Geometry check sheet. Reference: the model listing, model coordinates, mm. A direction names the side the tool comes from. Give positions to 0.01 mm unless a question says otherwise; leave off trailing zeros. Order: outer loops, then holes, each group sorted by start corner. A loop starts at its lowest first (then second) coordinate and runs counter-clockwise, first axis right, second up. Notation, with made-up numbers: M 36.5,85.25 L 78.5,85.25 A9 cw 78.5,94.25 Z; hole C 3.25,68.5 d2. An arc over 180 degrees is marked long. Answer as CSV lines item,"result". Start each with the question number.
```python
from build123d import *

# Parameters (mm, degrees)
SKETCH_1_W               = 28
SKETCH_1_H               = 64
EXTRUDE_1_DEPTH          = 74
SKETCH_2_R               = 2.5
CUT_EXTRUDE_1_DEPTH      = 10
CUT_EXTRUDE_2_DEPTH      = 99.833192805
CUT_EXTRUDE_2_DEPTH_BACK = 99.833192805
SKETCH_3_W               = 54
SKETCH_3_H               = 40
EXTRUDE_2_DEPTH          = 80
SKETCH_6_R               = 10.5
CUT_EXTRUDE_3_DEPTH      = 123.719191653
SKETCH_11_W              = 28
SKETCH_11_H              = 5
SKETCH_11_H_2            = 4
EXTRUDE_5_DEPTH          = 67
SKETCH_12_R              = 2
CUT_EXTRUDE_8_DEPTH      = 122.231184107
CHAMFER_1_SIZE           = 10
SKETCH_13_R              = 10.5
SKETCH_13_R_2            = 9.5
EXTRUDE_6_DEPTH          = 25
SKETCH_14_R              = 2
CUT_EXTRUDE_9_DEPTH      = 119.894911582
SKETCH_15_R              = 2
CUT_EXTRUDE_10_DEPTH     = 122.342490596
CHAMFER_2_SIZE           = 3


with BuildPart() as part:
    # 草图1 → 凸台-拉伸1 (new body)
    with BuildSketch(Plane.XY):
        with Locations((0, 32)):
            Rectangle(SKETCH_1_W, SKETCH_1_H)
    extrude(amount=EXTRUDE_1_DEPTH)

    # 草图2 → 切除-拉伸1 (cut)
    with BuildSketch(Plane.XY.offset(74)):
        with Locations((-8, 58)):
            Circle(SKETCH_2_R)
        with Locations((8, 58)):
            Circle(SKETCH_2_R)
        with Locations((-8, 6)):
            Circle(SKETCH_2_R)
        with Locations((8, 6)):
            Circle(SKETCH_2_R)
    extrude(amount=-CUT_EXTRUDE_1_DEPTH, mode=Mode.SUBTRACT)

    # 草图3 → 切除-拉伸2 (cut, two sides: drawn at the far end of the back side and taken through both)
    with BuildSketch(Plane(origin=(0, 0, 0), x_dir=(0, 0, -1), z_dir=(1, 0, 0)).offset(-CUT_EXTRUDE_2_DEPTH_BACK)):
        with Locations((-37, 32)):
            Rectangle(SKETCH_3_W, SKETCH_3_H)
    extrude(amount=CUT_EXTRUDE_2_DEPTH + CUT_EXTRUDE_2_DEPTH_BACK, mode=Mode.SUBTRACT)

    # 草图4 → 凸台-拉伸2 (add)
    with BuildSketch(Plane(origin=(0, 0, 37), x_dir=(-1, 0, 0), z_dir=(0, 0, -1))):
        with BuildLine():
            Line((-14, 2), (14, 2))
            Line((14, 2), (14, -14))
            ThreePointArc((14, -14), (0, -28), (-14, -14))
            Line((-14, -14), (-14, 2))
        make_face()
        with BuildLine():
            Line((14, 62), (14, 78))
            ThreePointArc((14, 78), (0, 92), (-14, 78))
            Line((-14, 78), (-14, 62))
            Line((-14, 62), (14, 62))
        make_face()
    extrude(amount=EXTRUDE_2_DEPTH)

    # 草图6 → 切除-拉伸3 (cut, through all)
    with BuildSketch(Plane(origin=(0, 0, 37), x_dir=(-1, 0, 0), z_dir=(0, 0, -1))):
        with Locations((0, -14)):
            Circle(SKETCH_6_R)
        with Locations(Location((0, 78, 0), (0, 0, 180))):
            Circle(SKETCH_6_R)
    extrude(amount=CUT_EXTRUDE_3_DEPTH, mode=Mode.SUBTRACT)

    # 草图11 → 凸台-拉伸5 (add)
    with BuildSketch(Plane(origin=(0, 0, 0), x_dir=(-1, 0, 0), z_dir=(0, 0, -1))):
        with Locations((0, 64.5)):
            Rectangle(SKETCH_11_W, SKETCH_11_H)
        Rectangle(SKETCH_11_W, SKETCH_11_H_2)
    extrude(amount=EXTRUDE_5_DEPTH)

    # 草图12 → 切除-拉伸8 (cut, through all)
    with BuildSketch(Plane(origin=(0, 67, 0), x_dir=(1, 0, 0), z_dir=(0, 1, 0))):
        with Locations(Location((-9, 62, 0), (0, 0, 270))):
            Circle(SKETCH_12_R)
        with Locations(Location((9, 62, 0), (0, 0, 270))):
            Circle(SKETCH_12_R)
    extrude(amount=-CUT_EXTRUDE_8_DEPTH, mode=Mode.SUBTRACT)

    # 倒角1
    chamfer_1_edges = [part.edges().sort_by_distance(p)[0] for p in [
        (0, 62, 0),
        (0, 2, 0),
    ]]
    chamfer(chamfer_1_edges, length=CHAMFER_1_SIZE)

    # 草图13 → 凸台-拉伸6 (add, symmetric)
    # profile 1 of 2: a face of its own
    with BuildSketch(Plane.XY.offset(-3)):
        with Locations((0, 78)):
            Circle(SKETCH_13_R)
        with Locations((0, 78)):
            Circle(SKETCH_13_R_2, mode=Mode.SUBTRACT)
    # profile 2 of 2: a face of its own
    with BuildSketch(Plane.XY.offset(-3)):
        with Locations(Location((0, -14, 0), (0, 0, 180))):
            Circle(SKETCH_13_R)
        with Locations(Location((0, -14, 0), (0, 0, 180))):
            Circle(SKETCH_13_R_2, mode=Mode.SUBTRACT)
    extrude(amount=EXTRUDE_6_DEPTH, both=True)

    # 草图14 → 切除-拉伸9 (cut, through all)
    with BuildSketch(Plane(origin=(0, 0, 0), x_dir=(0, 0, -1), z_dir=(1, 0, 0))):
        with Locations((-29, 78)):
            Circle(SKETCH_14_R)
        with Locations((35, 78)):
            Circle(SKETCH_14_R)
        with Locations((35, -14)):
            Circle(SKETCH_14_R)
        with Locations((-29, -14)):
            Circle(SKETCH_14_R)
    extrude(amount=-CUT_EXTRUDE_9_DEPTH, mode=Mode.SUBTRACT)

    # 草图15 → 切除-拉伸10 (cut, through all)
    with BuildSketch(Plane.ZY.offset(14)):
        with Locations(Location((34, 58, 0), (0, 0, 270))):
            Circle(SKETCH_15_R)
    extrude(amount=-CUT_EXTRUDE_10_DEPTH, mode=Mode.SUBTRACT)

    # 倒角2
    chamfer_2_edges = [part.edges().sort_by_distance(p)[0] for p in [
        (-9, -2, -64),
        (-9, 67, -64),
        (9, -2, -64),
        (9, 67, -64),
    ]]
    chamfer(chamfer_2_edges, length=CHAMFER_2_SIZE - 0.0001)  # a hair under: the kernel refuses the full size


solid = part.part
```
Item 1: Section check A-A on z = 25.5. Record the boundary of the cut face in (x, y), then the cut area to 3 significant figures.
Item 2: Depth check by flat-ended pin: pin 1 Ø6 at (x, z) = (10.5, 32) entering from -Y; pin 2 Ø15 at (x, y) = (0, 78) entering from -Z; pin 3 Ø14 at (x, y) = (-5, 23) entering from -Z; pin 4 Ø8.5 at (x, z) = (2.5, 49.5) entering from +Y. Enter the tip coordinate at first touch or a pass-through.
Item 3: Section check D-D on x = 0. Give the number of separate pieces and of enclosed holes in the cut face, then the cut area to 3 significant figures.
Item 4: Draft check along Y on faces 4 (the face through (0, -3, -43)), 5 (the face through (0, 92, -2)), 6 (the face through (-12.128, 78.601, 27.092)). Enter one of: pulls with the +Y half, pulls with the -Y half, needs draft (parallel to the pull), parting line crosses it, or undercut.
Item 5: Section check B-B on y = 32. Record the boundary of the cut face in (x, z).
Item 6: Access from +Z, -Z, +X, -X, +Y, -Y to the whole of each face (thin tool, end or side, straight path). Record for faces 1 (the face through (10.385, 6.751, 69.07)), 2 (the face through (0, 57, -5)), 3 (the face through (0, 0, 55)).
Item 7: Section check C-C on z = -45. Record the boundary of the cut face in (x, y).
Item 8: Scan lines: line 1 along Y through (x, z) = (0, -21.5); line 2 along Z through (x, y) = (-11.8, -14); line 3 along Y through (x, z) = (8, 68.75). Record each from-to range of solid material in increasing order.
Numbers:
1,outline,"M -14,-14 A14 ccw 14,-14 L 14,12 L -14,12 Z; M -14,52 L 14,52 L 14,78 A14 ccw -14,78 Z; hole C 0,-14 d21; hole C 0,78 d21"
1,area,"1,380 mm2"
2,pin 1,"y = -25.82"
2,pin 2,"through"
2,pin 3,"z = 0"
2,pin 4,"y = 64"
3,separate pieces,"3"
3,enclosed holes,"2"
3,area,"4,370 mm2"
4,face 4,"needs draft"
4,face 5,"pulls with the +Y half"
4,face 6,"undercut"
5,outline,"M -14,0 L 14,0 L 14,10 L -14,10 Z; M -14,64 L 14,64 L 14,74 L -14,74 Z"
6,face 1,"+Z"
6,face 2,"-Z, +X, -X"
6,face 3,"+Z, +X, -X, -Y"
7,outline,"M -14,-2 L 14,-2 L 14,2 L -14,2 Z; M -14,62 L 14,62 L 14,67 L -14,67 Z"
8,line 1,"-28 to -23.5, -4.5 to 2, 62 to 68.5, 87.5 to 92"
8,line 2,"-43 to -37, -33 to 27, 31 to 37"
8,line 3,"0 to 3.5, 8.5 to 55.5, 60.5 to 64"
